For this review, take the finished solid that the model builds, in its own axes (mm). Face numbers are marked on the shaded views. A direction names the side the tool comes from. Give positions to 0.01 mm unless a question says otherwise; leave off trailing zeros. Order: outer loops, then holes, each group sorted by start corner. A loop starts at its lowest first (then second) coordinate and runs counter-clockwise, first axis right, second up.
from build123d import *

# Parameters (mm, degrees)
F2_DEPTH = 46
F3_W     = 30
F3_H     = 46
F4_DEPTH = 6.001


with BuildPart() as f2:
    # F1 (on Right) → F2 (new body)
    with BuildSketch(Plane.YZ):
        Polygon((-9, 38), (-6, 38), (-6, 3), (-12, 3), (-12, -5), (-9, -5), (-9, 0), (-3, 0), (-3, 41), (-12, 41), (-12, 33), (-9, 33), align=None)
    extrude(amount=F2_DEPTH)

    # F3 (on face) → F4 (cut, through all)
    with BuildSketch(Plane.XZ.offset(6)):
        with Locations((23, 18)):
            Rectangle(F3_W, F3_H)
    extrude(amount=F4_DEPTH, mode=Mode.SUBTRACT)


solid = f2.part
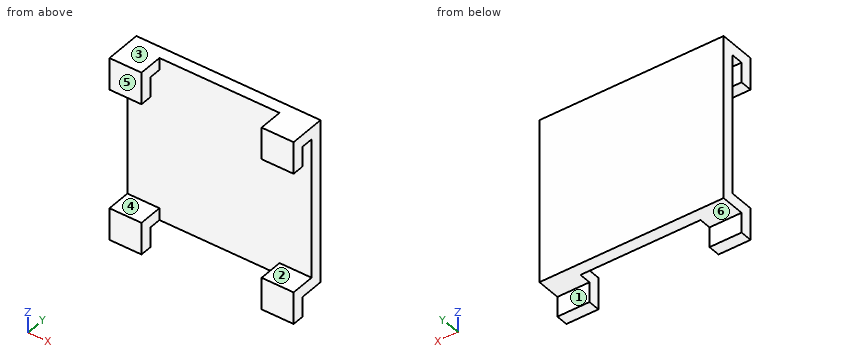
1) We need section A-A on z = 36.5. Give the boundary of the cut face in (x, y), then the cut area to 3 significant figures.
Answer sheet:
outline: (0, -12) - (8, -12) - (8, -9) - (0, -9) - close; (0, -6) - (46, -6) - (46, -3) - (0, -3) - close; (38, -12) - (46, -12) - (46, -9) - (38, -9) - close
area: 186 mm2
2) We need section D-D on z = 1. Give the boundary of the cut face in (x, y), then the cut area to 3 significant figures.
Answer sheet:
outline: (0, -12) - (8, -12) - (8, -6) - (38, -6) - (38, -12) - (46, -12) - (46, -3) - (0, -3) - close
area: 234 mm2
3) We need section B-B on y = -7.5. Give the boundary of the cut face in (x, z), then the cut area to 3 significant figures.
Answer sheet:
outline: (0, 0) - (8, 0) - (8, 3) - (0, 3) - close; (0, 38) - (8, 38) - (8, 41) - (0, 41) - close; (38, 0) - (46, 0) - (46, 3) - (38, 3) - close; (38, 38) - (46, 38) - (46, 41) - (38, 41) - close
area: 96.0 mm2
4) Clearance check with flat-ended pins moving along their axes: pin 1 (0.9 mm diameter, centred on x = 43.5, y = -7, fed in from -Z); pin 2 (8 mm diameter, centred on x = 27, z = 29.5, fed in from -Y). State where each tip first meets the part, or that it passes through.
Answer sheet:
pin 1: stops at z = 0
pin 2: stops at y = -6
5) Draft analysis for pull direction Z (two halves, no side actions). For the marked faces 4, 5 and 6, state which applies: +Z half, -Z half, draft (parallel to the pull), parting line (faces both ways), or undercut.
Answer sheet:
face 4: undercut
face 5: draft
face 6: -Z half
6) We need section C-C on x = 6. Give the boundary of the cut face in (y, z), then the cut area to 3 significant figures.
Answer sheet:
outline: (-12, -5) - (-9, -5) - (-9, 0) - (-3, 0) - (-3, 41) - (-12, 41) - (-12, 33) - (-9, 33) - (-9, 38) - (-6, 38) - (-6, 3) - (-12, 3) - close
area: 189 mm2
7) Tool access review of the marked faces 1, 2 and 3: name each direction out of +Z, -Z, +X, -X, +Y, -Y from which nothing blocks a thin tool from reaching the whole face with its end or side.
Answer sheet:
face 1: -Z, +X, -X, +Y
face 2: +X, -X, -Y
face 3: +Z, +X, -X, +Y, -Y
8) To check wall thickness, follow line 1 (Z direction, x = 7, y = -11.25); line 2 (Y direction, x = 9, z = 6); line 3 (Z direction, x = 17.5, y = -3.75). State the ranges of each line that lie inside material, in increasing order.
Answer sheet:
line 1: z = -5 to 3, 33 to 41
line 2: y = -6 to -3
line 3: z = 0 to 41
